Source: CAD feature listing. Evaluate the final solid. Frame: model axes, mm. Face numbers are marked on the shaded views. A direction names the side the tool comes from. Coordinates: 2 decimals unless noted, no trailing zeros. Write each loop counter-clockwise with the first axis right and the second up, starting at its lowest first coordinate (ties: lowest second). Pieces come first, ordered by that corner, then holes. Notation, with made-up numbers: (86, 64.5) - (100, 64.5) arc R32 ccw to (100, 94.5) - close; hole circle Ø6 at (-32.5, 72.25). An arc over 180 degrees is marked (long way). One line per question, with ' | ' between items. Start each with the question number.
Q1. Cut plane A-A, the plane z = 6.5. Give the number of separate pieces and of enclosed holes in the cut face, plus the area to 3 significant figures.
Q2. Draft query along X for the marked faces 4, 5 and 6. Return one class per face: +X half, -X half, draft (parallel to the pull), parting line (faces both ways), or undercut.
Q3. Contact query for flat-ended pins moving along their axis: P1, Ø4.5, axis at y = -5.5, z = 29.5, coming from the -X side; P2, Ø4, axis at x = 34.5, z = 1.5, coming from the +Y side; P3, Ø6.5, axis at y = -7, z = 22.5, coming from the -X side. Output: stop coordinate, or through.
Q4. Access query for the marked faces 1, 2 and 3. Directions: +Z, -Z, +X, -X, +Y, -Y. A direction counts if a zero-diameter tool reaches every point of the face in a straight line with its end or side. Return the directions, or none.
Q5. Cut plane D-D, the plane x = -31. Return loops of the section in (y, z).
Q6. Cut plane B-B, the plane y = -31. Return loops of the section in (x, z).
Q7. Line query: line 1 (X direction, y = -22.5, z = 10.5); line 2 (Y direction, x = 28.5, z = 8); line 3 (Y direction, x = 23, z = 7). Output: solid intervals per line, ascending.
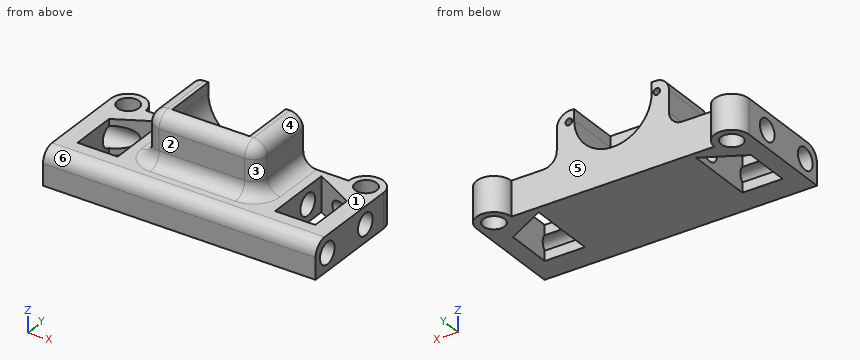
```python
from build123d import *

# Parameters (mm, degrees)
F0_R      = 4.025
F1_DEPTH  = 13
F2_R      = 4.05
F3_DEPTH  = 120
F5_DEPTH  = 18
F6_R      = 1.25
F7_DEPTH  = 20
F8_R      = 4.99999
F10_DEPTH = 25


# Not quite as in the source:
# - a fillet or chamfer is up to 0.001 mm smaller than in the source, because OpenCascade refuses the exact size


with BuildPart() as f1:
    # F0 (on Top) → F1 (new body)
    with BuildSketch(Plane.XY):
        with BuildLine():
            Line((38, 0), (0, 0))
            Line((0, 0), (-38, 0))
            ThreePointArc((-38, 0), (-44.5, 6.5), (-51, 0))
            Line((-51, 0), (-51, -37.5))
            Line((-51, -37.5), (0, -37.5))
            Line((0, -37.5), (51, -37.5))
            Line((51, -37.5), (51, 0))
            ThreePointArc((51, 0), (44.5, 6.5), (38, 0))
        make_face()
        with Locations((-44.5, 0)):
            Circle(F0_R, mode=Mode.SUBTRACT)
        with Locations((44.5, 0)):
            Circle(F0_R, mode=Mode.SUBTRACT)
    extrude(amount=F1_DEPTH)

    # F2 (on face) → F3 (cut)
    with BuildSketch(Plane.YZ.offset(51)):
        with Locations((-31, 6.5)):
            Circle(F2_R)
        with Locations((-10, 6.5)):
            Circle(F2_R)
    extrude(amount=-F3_DEPTH, mode=Mode.SUBTRACT)

    # F4 (on face) → F5 (join)
    with BuildSketch(Plane.XY.offset(13)):
        Polygon((-21, -25), (0, -25), (21, -25), (21, 0), (-21, 0), align=None)
    extrude(amount=F5_DEPTH)

    # F6 (on face) → F7 (cut)
    with BuildSketch(Plane(origin=(0, 0, 0), x_dir=(-1, 0, 0), z_dir=(0, 1, 0))):
        with BuildLine():
            Line((-14.5, 31), (-14.5, 27))
            ThreePointArc((-14.5, 27), (0, 12.5), (14.5, 27))
            Line((14.5, 27), (14.5, 31))
            Line((14.5, 31), (-14.5, 31))
        make_face()
        with Locations((-16.4399370551, 27)):
            Circle(F6_R)
        with Locations((16.4399370551, 27)):
            Circle(F6_R)
    extrude(amount=-F7_DEPTH, mode=Mode.SUBTRACT)

    # F8 (radius 5 in the source; OpenCascade refuses exactly that, so slightly less here)
    f8_edges = [f1.edges().sort_by_distance(p)[0] for p in [
        (21, -12.5, 31),
        (-21, -12.5, 31),
        (21, -12.5, 13),
        (-21, -12.5, 13),
        (0, -25, 31),
        (21, -25, 22),
        (-21, -25, 22),
        (0, -37.5, 13),
        (0, -25, 13),
    ]]
    fillet(f8_edges, radius=F8_R)

    # F9 (on face) → F10 (cut)
    with BuildSketch(Plane.XY.offset(13)):
        Polygon((44.5, -28.0575975776), (44.5, -10.6131481007), (29.4615291059, -2.4116530549), (29.4615291059, -28.0575975776), align=None)
        Polygon((-29.4615291059, -2.4116530549), (-44.5, -10.6131481007), (-44.5, -28.0575975776), (-29.4615291059, -28.0575975776), align=None)
    extrude(amount=-F10_DEPTH, mode=Mode.SUBTRACT)


solid = f1.part
```
Reply:
1) separate pieces: 5 | enclosed holes: 2 | area: 1,790 mm^2
2) face 4: +X half | face 5: undercut | face 6: draft
3) P1: stops at x = -20.84 | P2: stops at y = 0 | P3: stops at x = -21
4) face 1: +Z, -Y | face 2: +Z, +X, -X, -Y | face 3: +Z, +X, -Y
5) outline: (-37.5, 0) - (-28.06, 0) - (-28.06, 3.72) arc R4.05 cw (long way) to (-28.06, 9.28) - (-28.06, 13) - (-32.5, 13) arc R5 ccw to (-37.5, 8) - close; (-3.25, 0) - (0, 0) - (0, 13) - (-3.25, 13) - close
6) outline: (-51, 0) - (51, 0) - (51, 2.45) - (-51, 2.45) - close; (-51, 10.55) - (51, 10.55) - (51, 13) - (-51, 13) - close
7) line 1: x = -51 to -44.5, -29.46 to 29.46, 44.5 to 51 | line 2: y = -37.5 to -34.76, -27.24 to -13.76, -6.24 to 0 | line 3: y = -37.5 to -35.02, -26.98 to -14.02, -5.98 to 0
